from build123d import *

# Parameters (mm, degrees)
F1_DEPTH = 200


with BuildPart() as f1:
    # F0 (on Front) → F1 (new body, symmetric)
    with BuildSketch(Plane.XZ):
        with BuildLine():
            Line((0, 150), (0, 140))
            ThreePointArc((0, 140), (-10.990919, 139.567904), (-21.913993, 138.274282))
            Line((-21.913993, 138.274282), (-23.441789, 147.920408))
            ThreePointArc((-23.441789, 147.920408), (-34.968111, 145.508317), (-46.269651, 142.199316))
            Line((-46.269651, 142.199316), (-43.322337, 133.128416))
            ThreePointArc((-43.322337, 133.128416), (-53.673121, 129.30273), (-63.690435, 124.673688))
            Line((-63.690435, 124.673688), (-67.921488, 132.977595))
            ThreePointArc((-67.921488, 132.977595), (-78.138294, 127.121731), (-87.86416, 120.482316))
            Line((-87.86416, 120.482316), (-82.50488, 113.105901))
            ThreePointArc((-82.50488, 113.105901), (-91.18094, 106.235757), (-99.287246, 98.701787))
            Line((-99.287246, 98.701787), (-105.606612, 105.021153))
            ThreePointArc((-105.606612, 105.021153), (-113.51381, 96.294728), (-120.711966, 86.974812))
            Line((-120.711966, 86.974812), (-113.607356, 81.81301))
            ThreePointArc((-113.607356, 81.81301), (-119.727162, 72.563122), (-125.095543, 62.857817))
            Line((-125.095543, 62.857817), (-132.808279, 66.787653))
            ThreePointArc((-132.808279, 66.787653), (-137.631858, 56.04487), (-141.597698, 44.956751))
            Line((-141.597698, 44.956751), (-133.453437, 42.31052))
            ThreePointArc((-133.453437, 42.31052), (-136.387276, 31.599222), (-138.462855, 20.689076))
            Line((-138.462855, 20.689076), (-146.8638, 22.019655))
            ThreePointArc((-146.8638, 22.019655), (-148.131594, 10.312094), (-148.476915, -1.458846))
            Line((-148.476915, -1.458846), (-139.992399, -1.458846))
            ThreePointArc((-139.992399, -1.458846), (-139.435962, -12.554384), (-138.001501, -23.570867))
            Line((-138.001501, -23.570867), (-146.397324, -24.900635))
            ThreePointArc((-146.397324, -24.900635), (-143.985232, -36.426957), (-140.676231, -47.728497))
            Line((-140.676231, -47.728497), (-132.541707, -45.085429))
            ThreePointArc((-132.541707, -45.085429), (-128.552613, -55.4457), (-123.755159, -65.457318))
            Line((-123.755159, -65.457318), (-131.454511, -69.380334))
            ThreePointArc((-131.454511, -69.380334), (-125.598646, -79.59714), (-118.959231, -89.323006))
            Line((-118.959231, -89.323006), (-111.870329, -84.172617))
            ThreePointArc((-111.870329, -84.172617), (-104.861356, -92.758267), (-97.195184, -100.762573))
            Line((-97.195184, -100.762573), (-103.498068, -107.065458))
            ThreePointArc((-103.498068, -107.065458), (-94.771643, -114.972656), (-85.451727, -122.170812))
            Line((-85.451727, -122.170812), (-80.108083, -114.815918))
            ThreePointArc((-80.108083, -114.815918), (-70.798197, -120.779201), (-61.046779, -125.989248))
            Line((-61.046779, -125.989248), (-65.264568, -134.267125))
            ThreePointArc((-65.264568, -134.267125), (-54.467372, -139.112599), (-43.321732, -143.09164))
            ThreePointArc((-43.321732, -143.09164), (2.292038, -145.364646), (46.028998, -132.216986))
            ThreePointArc((46.028998, -132.216986), (56.22186, -128.215063), (66.070765, -123.428741))
            Line((66.070765, -123.428741), (70.903418, -132.913357))
            ThreePointArc((70.903418, -132.913357), (81.120225, -127.057492), (90.84609, -120.418077))
            Line((90.84609, -120.418077), (84.471787, -111.644602))
            ThreePointArc((84.471787, -111.644602), (92.915532, -104.722032), (100.794109, -97.162481))
            Line((100.794109, -97.162481), (108.588542, -104.956914))
            ThreePointArc((108.588542, -104.956914), (116.495741, -96.230489), (123.693897, -86.910573))
            Line((123.693897, -86.910573), (114.652585, -80.341675))
            ThreePointArc((114.652585, -80.341675), (120.552663, -71.183252), (125.722736, -61.59378))
            Line((125.722736, -61.59378), (135.790209, -66.723414))
            ThreePointArc((135.790209, -66.723414), (140.613788, -55.980632), (144.579629, -44.892512))
            Line((144.579629, -44.892512), (133.747113, -41.372814))
            ThreePointArc((133.747113, -41.372814), (136.555986, -30.861994), (138.540179, -20.164793))
            Line((138.540179, -20.164793), (149.845731, -21.955417))
            ThreePointArc((149.845731, -21.955417), (151.113525, -10.247856), (151.458846, 1.523085))
            Line((151.458846, 1.523085), (139.991715, 1.523085))
            ThreePointArc((139.991715, 1.523085), (139.451051, 12.385652), (138.068788, 23.173472))
            Line((138.068788, 23.173472), (149.379254, 24.964874))
            ThreePointArc((149.379254, 24.964874), (146.967163, 36.491196), (143.658162, 47.792735))
            Line((143.658162, 47.792735), (132.816291, 44.269998))
            ThreePointArc((132.816291, 44.269998), (128.975931, 54.453735), (124.356076, 64.308369))
            Line((124.356076, 64.308369), (134.436441, 69.444572))
            ThreePointArc((134.436441, 69.444572), (128.580576, 79.661379), (121.941162, 89.387244))
            Line((121.941162, 89.387244), (112.884668, 82.807316))
            ThreePointArc((112.884668, 82.807316), (106.098821, 91.340244), (98.669568, 99.319265))
            Line((98.669568, 99.319265), (106.479999, 107.129696))
            ThreePointArc((106.479999, 107.129696), (97.753574, 115.036895), (88.433658, 122.235051))
            Line((88.433658, 122.235051), (82.044101, 113.440581))
            ThreePointArc((82.044101, 113.440581), (72.944753, 119.495034), (63.400833, 124.82121))
            Line((63.400833, 124.82121), (68.246499, 134.331363))
            ThreePointArc((68.246499, 134.331363), (57.503716, 139.154943), (46.415597, 143.120783))
            Line((46.415597, 143.120783), (43.183531, 133.173506))
            ThreePointArc((43.183531, 133.173506), (32.630677, 136.144184), (21.877732, 138.280023))
            Line((21.877732, 138.280023), (23.478501, 148.386885))
            ThreePointArc((23.478501, 148.386885), (11.77094, 149.654679), (0, 150))
        make_face()
        with BuildLine():
            ThreePointArc((0, 25), (17.67767, 17.67767), (25, 0))
            ThreePointArc((25, 0), (-17.67767, -17.67767), (0, 25))
        make_face(mode=Mode.SUBTRACT)
        with BuildLine():
            ThreePointArc((46.028998, -132.216986), (2.292038, -145.364646), (-43.321732, -143.09164))
            Line((-43.321732, -143.09164), (-56.696378, -186.051216))
            Line((-56.696378, -186.051216), (-80.108083, -186.051216))
            Line((-80.108083, -186.051216), (-80.108083, -206.051216))
            Line((-80.108083, -206.051216), (84.471787, -206.051216))
            Line((84.471787, -206.051216), (84.471787, -186.051216))
            Line((84.471787, -186.051216), (64.606167, -186.051216))
            Line((64.606167, -186.051216), (46.028998, -132.216986))
        make_face()
    extrude(amount=F1_DEPTH, both=True)


solid = f1.part
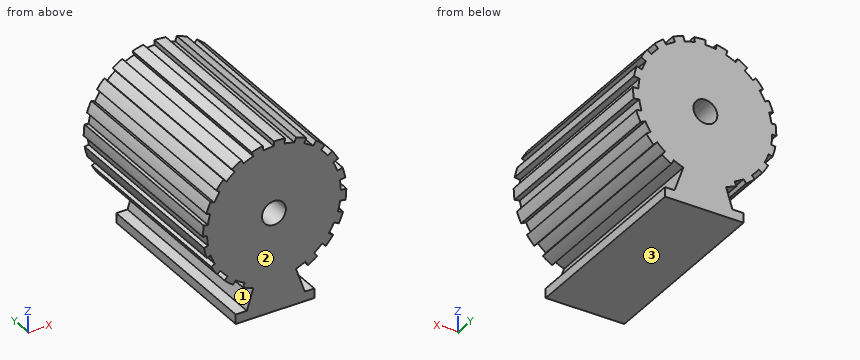
Work out the finished part from the listing and answer in its coordinate system (mm). Face numbers are marked on the shaded views. Give positions to 0.01 mm unless a question says otherwise; leave off trailing zeros. Order: outer loops, then holes, each group sorted by start corner. A loop starts at its lowest first (then second) coordinate and runs counter-clockwise, first axis right, second up. Notation, with made-up numbers: M -17,67 L 35,67 A19 cw 35,93 Z; hole C -32.75,50.5 d1. An arc over 180 degrees is marked long. Return JSON: item names as keys, results as strings.
Q1. Find the intervals of material crossed by line 1 along X through (y, z) = (96, 0); line 2 along Z through (x, y) = (-68, 170.5); line 3 along Z through (x, y) = (106, 152), in increasing order. Write a range as [from, to].
Answer below:
{"line 1": "x = [-148.48, -25], [25, 151.47]", "line 2": "z = [-206.05, -186.05], [-122.38, 132.94]", "line 3": "z = [-102.37, 91.45], [106.65, 107.6]"}
Q2. The mould has two halves that part along Z. Classify the marked faces 1, 2 and 3: pulls with the +Z half, pulls with the -Z half, needs draft (parallel to the pull), parting line crosses it, or undercut.
Answer below:
{"face 1": "undercut", "face 2": "needs draft", "face 3": "pulls with the -Z half"}
Q3. Find section A-A, the plane x = -5.5. Write down the section's boundary in (y, z).
Answer below:
{"outline": "M -200,-206.05 L 200,-206.05 L 200,-24.39 L -200,-24.39 Z; M -200,24.39 L 200,24.39 L 200,139.89 L -200,139.89 Z"}
Q4. Each of these flat-tipped pins is pushed along its axis until it touches: pin 1 (6 mm diameter, centred on y = -61, z = -199, fed in from +X); pin 2 (6 mm diameter, centred on x = -48, y = 28, fed in from +Z); pin 3 (4 mm diameter, centred on y = 104.5, z = -136.5, fed in from -X). Where does it stop, or does it pass through?
Answer below:
{"pin 1": "stops at x = 84.47", "pin 2": "stops at z = 142.62", "pin 3": "stops at x = -64.79"}
